Build history of the part. All positions in model axes, mm. A direction names the side the tool comes from. Give positions to 0.01 mm unless a question says otherwise; leave off trailing zeros. Order: outer loops, then holes, each group sorted by start corner. A loop starts at its lowest first (then second) coordinate and runs counter-clockwise, first axis right, second up. Notation, with made-up numbers: M 76,57 L 116,57 A22 cw 116,85 Z; hole C 42,-21 d5. An arc over 180 degrees is marked long. Use CSV: the item, a comma, the result in double quotes. Start each with the question number.
Item 1: Two-plate mould, pull along X, no slides. Class faces 1 (the flat face through (38, 16, 10)), 2 (the flat face through (43, 3, 10)), 3 (the flat face through (14, 32, 9)), 4 (the flat face through (38, 3, 10)): pulls with the +X half, pulls with the -X half, needs draft (parallel to the pull), parting line crosses it, or undercut.
Item 2: Band-saw the part on A-A on x = 15. Write the cut outline in (y, z).
Item 3: Which spindle directions (+Z, -Z, +X, -X, +Y, -Y) get a long thin tool onto all of the face, cutting with end or side? Do faces 5 (the flat face through (30, 13.5, 10)), 6 (the cylindrical face through (29.182, 18.199, 19.715)), 7 (the flat face through (17, 25, 10)), 8 (the cylindrical face through (16.699, 9.176, 19.715)). Say none if no direction does.
Item 4: Band-saw the part on B-B on y = 7. Write the cut outline in (x, z), plus the area to 3 significant figures.
Item 5: Band-saw the part on C-C on x = 31.5. Write the cut outline in (y, z), plus the area to 3 significant figures.
Item 6: Pin check, flat tips, straight feed: P1, Ø4, axis at y = 21, z = 12.5, coming from the +X side; P2, Ø4.5, axis at y = 2, z = 9, coming from the -X side; P3, Ø1, axis at x = 5, z = 14.5, coming from the +Y side. Stop position of each tip, or through.
Item 7: Wall check: line 1 along Y through (x, z) = (31, 5); line 2 along X through (y, z) = (19, 2); line 3 along X through (y, z) = (22.5, 9.75). Give the ranges that are in metal, low to high.
from build123d import *

# Parameters (mm, degrees)
PAD_DEPTH       = 20
FILLET_R        = 5
FILLET001_R     = 1
SKETCH001_W     = 5
SKETCH001_H     = 3
POCKET_DEPTH    = 31.001
FILLET002_R     = 0.5
SKETCH002_W     = 3
SKETCH002_H     = 5
POCKET001_DEPTH = 18.501
FILLET003_R     = 0.5


with BuildPart() as part:
    # Sketch → Pad (new body)
    with BuildSketch(Plane.XY):
        Polygon((5, 20), (5, 5), (12, 5), (12, 32), (17, 32), (17, 18.5), (43, 18.5), (43, 13.5), (17, 13.5), (17, 5), (43, 5), (43, 0), (0, 0), (0, 20), align=None)
    extrude(amount=PAD_DEPTH)

    # Fillet
    fillet_edges = [part.edges().sort_by_distance(p)[0] for p in [
        (0, 0, 10),
    ]]
    fillet(fillet_edges, radius=FILLET_R)

    # Fillet001
    fillet001_edges = [part.edges().sort_by_distance(p)[0] for p in [
        (0, 20, 10),
        (0, 12.5, 20),
        (0, 12.5, 0),
        (2.5, 20, 20),
        (2.5, 20, 0),
        (5, 20, 10),
        (12, 32, 10),
        (12, 18.5, 20),
        (8.5, 5, 20),
        (5, 12.5, 20),
        (17, 25.25, 20),
        (17, 32, 10),
        (30, 18.5, 0),
        (43, 18.5, 10),
        (30, 18.5, 20),
        (24, 0, 20),
        (1.464466, 1.464466, 20),
        (43, 2.5, 20),
        (30, 5, 20),
        (17, 9.25, 20),
        (30, 13.5, 20),
        (43, 16, 20),
        (14.5, 32, 20),
        (12, 18.5, 0),
        (17, 25.25, 0),
        (30, 13.5, 0),
        (17, 9.25, 0),
        (30, 5, 0),
        (8.5, 5, 0),
        (24, 0, 0),
        (43, 13.5, 10),
        (43, 16, 0),
        (43, 2.5, 0),
        (43, 0, 10),
        (43, 5, 10),
        (5, 12.5, 0),
    ]]
    fillet(fillet001_edges, radius=FILLET001_R)

    # Sketch001 (on Face47 of Fillet001) → Pocket (cut, through all)
    with BuildSketch(Plane(origin=(12, 0, 0), x_dir=(0, -1, 0), z_dir=(-1, 0, 0))):
        with Locations((-24.5, 5.5)):
            Rectangle(SKETCH001_W, SKETCH001_H)
        with Locations((-24.5, 14.5)):
            Rectangle(SKETCH001_W, SKETCH001_H)
    extrude(amount=-POCKET_DEPTH, mode=Mode.SUBTRACT)

    # Fillet002
    fillet002_edges = [part.edges().sort_by_distance(p)[0] for p in [
        (12, 22, 5.5),
        (12, 24.5, 16),
        (12, 27, 5.5),
        (12, 24.5, 4),
        (12, 24.5, 13),
        (12, 27, 14.5),
        (12, 5, 10),
        (12, 22, 14.5),
        (17, 27, 5.5),
        (17, 24.5, 16),
        (17, 22, 5.5),
        (17, 24.5, 4),
        (42.707107, 18.207107, 1),
        (17, 24.5, 7),
        (5, 5, 10),
        (42, 18.5, 10),
    ]]
    fillet(fillet002_edges, radius=FILLET002_R)

    # Sketch002 (on Face46 of Fillet002) → Pocket001 (cut, through all)
    with BuildSketch(Plane(origin=(0, 18.5, 0), x_dir=(-1, 0, 0), z_dir=(0, 1, 0))):
        with Locations((-36.5, 10)):
            Rectangle(SKETCH002_W, SKETCH002_H)
    extrude(amount=-POCKET001_DEPTH, mode=Mode.SUBTRACT)

    # Fillet003
    fillet003_edges = [part.edges().sort_by_distance(p)[0] for p in [
        (35, 18.5, 10),
        (36.5, 18.5, 7.5),
        (38, 18.5, 10),
        (36.5, 18.5, 12.5),
        (36.5, 5, 7.5),
        (38, 5, 10),
        (35, 5, 10),
        (36.5, 5, 12.5),
        (36.5, 0, 12.5),
        (35, 0, 10),
        (36.5, 0, 7.5),
        (38, 0, 10),
        (35, 13.5, 10),
        (36.5, 13.5, 12.5),
        (38, 13.5, 10),
        (36.5, 13.5, 7.5),
    ]]
    fillet(fillet003_edges, radius=FILLET003_R)


solid = part.part
Model answer:
1,face 1,"undercut"
1,face 2,"pulls with the +X half"
1,face 3,"needs draft"
1,face 4,"undercut"
2,outline,"M 0,1 A1 ccw 1,0 L 32,0 L 32,19 A1 ccw 31,20 L 1,20 A1 ccw 0,19 Z; hole M 22,4 L 27,4 L 27,7 L 22,7 Z; hole M 22,13 L 27,13 L 27,16 L 22,16 Z"
3,face 5,"+Z, -Z, +X"
3,face 6,"+Z, +X, +Y"
3,face 7,"+Z, -Z, +X, +Y"
3,face 8,"+Z, +X"
4,outline,"M 0,1 A1 ccw 1,0 L 4,0 A1 ccw 5,1 L 5,19 A1 ccw 4,20 L 1,20 A1 ccw 0,19 Z; M 12,1 A1 ccw 13,0 L 16,0 A1 ccw 17,1 L 17,19 A1 ccw 16,20 L 13,20 A1 ccw 12,19 Z"
4,area,"198 mm^2"
5,outline,"M 0,1 A1 ccw 1,0 L 4,0 A1 ccw 5,1 L 5,19 A1 ccw 4,20 L 1,20 A1 ccw 0,19 Z; M 13.5,1 A1 ccw 14.5,0 L 17.5,0 A1 ccw 18.5,1 L 18.5,19 A1 ccw 17.5,20 L 14.5,20 A1 ccw 13.5,19 Z"
5,area,"198 mm^2"
6,P1,"stops at x = 17"
6,P2,"stops at x = 0.06"
6,P3,"stops at y = 19.87"
7,line 1,"y = 0 to 5, 13.5 to 18.5"
7,line 2,"x = 0 to 5, 12 to 17"
7,line 3,"x = 12 to 17"
